```python
from build123d import *

# Parameters (mm, degrees)
SKETCH1_R               = 6
SKETCH1_R_2             = 1.475
BOSS_EXTRUDE1_DEPTH     = 4.5
CUT_EXTRUDE2_DEPTH      = 23.638462845
CUT_EXTRUDE2_DEPTH_BACK = 23.638462845
CUT_EXTRUDE1_START      = -6
CUT_EXTRUDE1_DEPTH      = 17.638462912
CHAMFER1_SIZE           = 2
CUT_EXTRUDE3_START      = 4.5
SKETCH9_R               = 6.5
CUT_EXTRUDE3_DEPTH      = 19.138462912
CUT_EXTRUDE4_START      = -4.5
SKETCH9_2_R             = 6.5
CUT_EXTRUDE4_DEPTH      = 19.138462913
SKETCH10_W              = 0.525
SKETCH10_H              = 0.5


with BuildPart() as part:
    # Sketch1 → Boss-Extrude1 (new, symmetric)
    with BuildSketch(Plane.XY):
        Circle(SKETCH1_R)
        Circle(SKETCH1_R_2, mode=Mode.SUBTRACT)
    extrude(amount=BOSS_EXTRUDE1_DEPTH, both=True)


with BuildPart() as body_2:
    # Sketch5 → Revolve1 (revolve)
    with BuildSketch(Plane.XY):
        with BuildLine():
            Line((0, -7.5), (-12.5, -7.5))
            ThreePointArc((-12.5, -7.5), (-17.803300859, -5.303300859), (-20, 0))
            Line((-20, 0), (0, 0))
            Line((0, 0), (0, -7.5))
        make_face()
    revolve(axis=Axis((-26.625188219, 0, 0), (1, 0, 0)))

    # Sketch7 → Cut-Extrude2 (cut, two sides: drawn at the far end of the back side and taken through both)
    with BuildSketch(Plane.XY.offset(-CUT_EXTRUDE2_DEPTH_BACK)):
        with BuildLine():
            Line((-3.652568574, -4.760120042), (-5.75495241, -7.5))
            Line((-5.75495241, -7.5), (0, -7.5))
            Line((0, -7.5), (0, -6))
            ThreePointArc((0, -6), (1.928636792, 5.681580777), (-3.652568574, -4.760120042))
        make_face()
    extrude(amount=CUT_EXTRUDE2_DEPTH + CUT_EXTRUDE2_DEPTH_BACK, mode=Mode.SUBTRACT)


with BuildPart() as part_1:
    add(part.part)

    # Combine1: union body 2
    add(body_2.part)

    # Sketch6 → Cut-Extrude1 (cut, through all)
    with BuildSketch(Plane(origin=(0, 0, 0), x_dir=(0, 0, -1), z_dir=(1, 0, 0)).offset(CUT_EXTRUDE1_START)):
        with BuildLine():
            ThreePointArc((-6, 4.5), (0, 5.752272915), (6, 4.5))
            ThreePointArc((6, 4.5), (0, 7.5), (-6, 4.5))
        make_face()
    extrude(amount=-CUT_EXTRUDE1_DEPTH, mode=Mode.SUBTRACT)

    # Chamfer1
    # the kernel refuses this chamfer: 2 mm, written as the material it adds along each edge
    with BuildSketch(Plane(origin=(-6, -9.247727085, 0), x_dir=(0, 0.7286512742865437, 0.6848848957895012), z_dir=(0, -0.6848848957895012, 0.7286512742865437))) as chamfer1_piece_1_section:
        Polygon((15, CHAMFER1_SIZE), (15 + CHAMFER1_SIZE, 0), (15, 0), align=None)
    chamfer1_piece_1 = revolve(axis=Axis((-6, -9.247727085, 0), (-1, 0, 0)), revolution_arc=86.453111056, mode=Mode.PRIVATE)
    chamfer1_piece_1 = chamfer1_piece_1 & Plane(origin=(-6.733016539, 0, 0), x_dir=(0, -1, 0), z_dir=(-1, 0, 0)) * Cylinder(7.5, 68, mode=Mode.PRIVATE)
    add(chamfer1_piece_1)

    # Sketch9 → Cut-Extrude3 (cut, through all)
    with BuildSketch(Plane.XY.offset(CUT_EXTRUDE3_START)):
        Circle(SKETCH9_R)
    extrude(amount=CUT_EXTRUDE3_DEPTH, mode=Mode.SUBTRACT)

    # Sketch9<2> → Cut-Extrude4 (cut, through all)
    with BuildSketch(Plane.XY.offset(CUT_EXTRUDE4_START)):
        Circle(SKETCH9_2_R)
    extrude(amount=-CUT_EXTRUDE4_DEPTH, mode=Mode.SUBTRACT)

    # Sketch10 → Revolve2 (revolve)
    with BuildSketch(Plane(origin=(0, 0, 0), x_dir=(1, 0, 0), z_dir=(0, 1, 0)), mode=Mode.PRIVATE) as revolve2_sk:
        with Locations((1.7375, 4.75)):
            Rectangle(SKETCH10_W, SKETCH10_H)
        with Locations((1.7375, -4.75)):
            Rectangle(SKETCH10_W, SKETCH10_H)
    revolve(revolve2_sk.sketch.rotate(Axis((0, 0, -4.5), (0, 0, 1)), 180), axis=Axis((0, 0, -4.5), (0, 0, 1)))


solid = part_1.part
```
Here's how the part is built. I have some questions about the finished solid (model axes, mm). A direction names the side the tool comes from. Give positions to 0.01 mm unless a question says otherwise; leave off trailing zeros. Order: outer loops, then holes, each group sorted by start corner. A loop starts at its lowest first (then second) coordinate and runs counter-clockwise, first axis right, second up. Notation, with made-up numbers: (36.5, 58.5) -> (75.5, 58.5) arc R33 cw to (75.5, 87.5) -> close; hole circle Ø9 at (-6, 70). An arc over 180 degrees is marked (long way). Use CSV: the item, a comma, the result in double quotes. Start each with the question number.
Item 1: On a 3-axis mill with a long thin cutter (end or side, diameter ignored), from which of +Z, -Z, +X, -X, +Y, -Y can I reach the whole of each face in a straight line? I mean faces 4 (the flat face through (-2, 1, -4.5)), 5 (the cylindrical face through (-12.593, 5.752, 0.086)), 6 (the flat face through (-4.46, -5.81, -0.08)). Say none if no direction works.
Item 2: If I drill on probe 1 along Y at (x, z) = (0, -4.85) (3 decimals); probe 2 along Y at (x, z) = (-11.5, 0.25); probe 3 along Z at (x, y) = (-0.5, 2.25), over which ranges is the centre line in solid material (lowest first)? Write a range as [from, to].
Item 3: Suppose I cut it at B-B (z = 0). List the corners of the cut face in (x, y) for me (3 decimals), and give its area (3 significant figures).
Item 4: Suppose I cut it at A-A (y = 0). List the corners of the cut face in (x, z) for me (3 decimals).
Item 5: I'm going to push flat-ended pins straight in: P1, Ø2, axis at x = -0.5, y = -0.5, coming from the -Z side; P2, Ø1.5, axis at x = -10, y = -3, coming from the +Z side; P3, Ø1, axis at x = -3, y = -5, coming from the +Z side; P4, Ø1.8, axis at x = 0, y = 0, coming from the +Z side. Where does each tip first touch, or does it pass through?
Item 6: Thinking about a two-plate mould opening in X: for faces 1 (the cylindrical face through (0.434, 1.952, 4.746)), 2 (the conical face through (-7.5, 6.25, 0.09)), 3 (the flat face through (0, 7, 0)), which applies, pulls with the +X half, pulls with the -X half, needs draft (parallel to the pull), parting line crosses it, or undercut?
Item 7: Suppose I cut it at D-D (y = -4). List the corners of the cut face in (x, z) for me, and give its area (3 significant figures).
Item 8: Suppose I cut it at C-C (x = -0.75). List the corners of the cut face in (y, z) for me, and give its area (3 significant figures).
Answer block:
1,face 4,"-Z"
1,face 5,"-X, +Y"
1,face 6,"+Z, -Z, -Y"
2,probe 1,"y = [-2, -1.475], [1.475, 2]"
2,probe 2,"y = [-7.5, 5.75]"
2,probe 3,"z = [-4.5, 4.5]"
3,outline,"(-17.313, 5.752) arc R7.5 ccw to (-12.5, -7.5) -> (-5.755, -7.5) -> (-3.653, -4.76) arc R6 ccw (long way) to (0, 6) -> (0, 7.5) -> (-6.252, 7.5) -> (-8, 5.752) -> close; hole circle Ø2.95 at (0, 0)"
3,area,"301 mm^2"
4,outline,"(-12.5, -7.5) -> (-6.5, -7.5) -> (-6.5, -4.5) -> (-2, -4.5) -> (-2, -5) -> (-1.475, -5) -> (-1.475, 5) -> (-2, 5) -> (-2, 4.5) -> (-6.5, 4.5) -> (-6.5, 7.5) -> (-12.5, 7.5) arc R7.5 ccw to start; (1.475, -5) -> (2, -5) -> (2, -4.5) -> (6, -4.5) -> (6, 4.5) -> (2, 4.5) -> (2, 5) -> (1.475, 5) -> close"
5,P1,"stops at z = -5"
5,P2,"stops at z = 7.15"
5,P3,"stops at z = 4.5"
5,P4,"passes through"
6,face 1,"undercut"
6,face 2,"pulls with the -X half"
6,face 3,"pulls with the +X half"
7,outline,"(-12.5, -6.34) -> (-5.12, -6.34) -> (-5.12, -4.5) -> (4.47, -4.5) -> (4.47, 4.5) -> (-5.12, 4.5) -> (-5.12, 6.34) -> (-12.5, 6.34) arc R6.34 ccw to start"
7,area,"243 mm^2"
8,outline,"(-5.95, -4.5) -> (-1.85, -4.5) -> (-1.85, -5) -> (-1.27, -5) -> (-1.27, 5) -> (-1.85, 5) -> (-1.85, 4.5) -> (-5.95, 4.5) -> close; (1.27, -5) -> (1.85, -5) -> (1.85, -4.5) -> (6, -4.5) arc R7.5 ccw to (6, 4.5) -> (1.85, 4.5) -> (1.85, 5) -> (1.27, 5) -> close"
8,area,"95.1 mm^2"
